from build123d import *

# Parameters (mm, degrees)
F0_R          = 4
F1_DEPTH      = 24.95
F2_W          = 40
F2_H          = 20
F3_DEPTH      = 150
F3_DEPTH_BACK = 150
F4_R          = 20
F5_DEPTH      = 50


with BuildPart() as f1:
    # F0 (on Top) → F1 (new body)
    with BuildSketch(Plane.XY):
        with BuildLine():
            Line((58.181364, 29.598313), (-78.941487, 29.598313))
            ThreePointArc((-78.941487, 29.598313), (-83.494247, 27.712498), (-85.380062, 23.159739))
            Line((-85.380062, 23.159739), (-85.380062, -34.03374))
            ThreePointArc((-85.380062, -34.03374), (-83.514933, -38.536559), (-79.012115, -40.401687))
            Line((-79.012115, -40.401687), (-73.01646, -40.401687))
            Line((-73.01646, -40.401687), (-58.498297, -40.401687))
            Line((-58.498297, -40.401687), (-46.752002, -40.401687))
            Line((-46.752002, -40.401687), (-43.284619, -40.401687))
            Line((-43.284619, -40.401687), (26.715381, -40.401687))
            Line((26.715381, -40.401687), (29.210588, -40.401687))
            Line((29.210588, -40.401687), (54.838952, -40.401687))
            Line((54.838952, -40.401687), (60.120346, -40.401687))
            ThreePointArc((60.120346, -40.401687), (63.302038, -39.083787), (64.619938, -35.902095))
            Line((64.619938, -35.902095), (64.619938, 23.159739))
            ThreePointArc((64.619938, 23.159739), (62.734124, 27.712498), (58.181364, 29.598313))
        make_face()
        with Locations((-77.880062, -32.901687)):
            Circle(F0_R, mode=Mode.SUBTRACT)
        with Locations((57.119938, -32.901687)):
            Circle(F0_R, mode=Mode.SUBTRACT)
        with Locations((-77.880062, 22.098313)):
            Circle(F0_R, mode=Mode.SUBTRACT)
        with Locations((57.119938, 22.098313)):
            Circle(F0_R, mode=Mode.SUBTRACT)
        Polygon((-58.498297, -40.401687), (-73.01646, -40.401687), (-46.752002, -66.558582), (-46.752002, -40.401687), align=None)
        Polygon((29.210588, -67.972728), (54.838952, -40.401687), (29.210588, -40.401687), align=None)
        Polygon((-46.752002, -40.401687), (-46.752002, -66.558582), (-46.752002, -82.901687), (-46.752002, -90.401687), (-39.252002, -90.401687), (21.710588, -90.401687), (29.210588, -90.401687), (29.210588, -82.901687), (29.210588, -67.972728), (29.210588, -40.401687), (26.715381, -40.401687), (-43.284619, -40.401687), align=None)
        with Locations((-39.252002, -82.901687)):
            Circle(F0_R, mode=Mode.SUBTRACT)
        with Locations((21.710588, -82.901687)):
            Circle(F0_R, mode=Mode.SUBTRACT)
    extrude(amount=-F1_DEPTH)

    # F2 (on face) → F3 (cut, two sides)
    with BuildSketch(Plane.YZ.offset(64.619938)) as f3_sk:
        with Locations((-5.902329, -10)):
            Rectangle(F2_W, F2_H)
    extrude(amount=-F3_DEPTH, mode=Mode.SUBTRACT)
    extrude(f3_sk.sketch, amount=-F3_DEPTH_BACK, mode=Mode.SUBTRACT)

    # F4 (on face) → F5 (cut)
    with BuildSketch(Plane.XZ.offset(90.401687)):
        with Locations((-8.770707, 0)):
            Circle(F4_R)
    extrude(amount=-F5_DEPTH, mode=Mode.SUBTRACT)


solid = f1.part
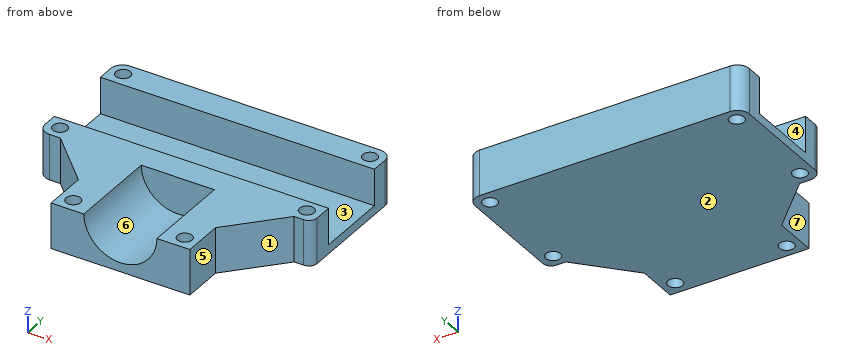
Verification items for the finished model (mm, model axes). Face numbers are marked on the shaded views. A direction names the side the tool comes from. Give positions to 0.01 mm unless a question says otherwise; leave off trailing zeros. Loops run counter-clockwise (first coordinate to the right, second up) from the corner with the lowest first, then second, coordinate; pieces in that order, holes last. Notation, with made-up numbers: (84, 55.25) - (99, 55.25) arc R16 cw to (99, 64.25) - close; hole circle Ø7 at (-25.75, 12.5). An arc over 180 degrees is marked (long way). Write item = value, one per line. Start each with the question number.
Q1. Thickness scan on line 1 (Y direction, x = 7, z = -18); line 2 (Y direction, x = -76, z = -7.25); line 3 (Y direction, x = -78.5, z = -20.75). Record the ranges inside material, lowest first.
Q2. Cross-section at C-C, the plane z = -23. Enter the section's corners in (x, y), and give its area (3 significant figures).
Q3. Depth check by flat-ended pin: P1, Ø6.5, axis at x = -39.25, y = -82.9, coming from the -Z side; P2, Ø2.5, axis at x = 57.5, z = -14, coming from the -Y side; P3, Ø4, axis at y = -48, z = -18.5, coming from the +X side; P4, Ø1.5, axis at y = -49, z = -11.5, coming from the -X side. Enter the tip coordinate at first touch or a pass-through.
Q4. Cross-section at B-B, the plane x = 16. Enter the section's corners in (y, z).
Q5. Tool access check on the marked faces 4, 5, 6 and 7. Record the directions out of +Z, -Z, +X, -X, +Y, -Y that give a thin tool (end or side, any length) a straight path to the whole face; none if there is none.
Q6. Cross-section at A-A, the plane z = -16. Enter the section's corners in (x, y), and give its area (3 significant figures).
Q7. Cross-section at D-D, the plane z = -6.5. Enter the section's corners in (x, y).
Q8. Mould release check, pull along Y, two halves, no side actions. Record for the marked faces 1, 2 and 3: released by +Y, released by -Y, zero draft, split by the parting line, or undercut.
Answer key:
q1.line_1 = -90.4 to -25.9, 14.1 to 29.6
q1.line_2 = -40.4 to -36.43, -29.37 to -25.9, 14.1 to 18.57, 25.63 to 29.6
q1.line_3 = -40.4 to -36.85, -28.95 to 18.15, 26.05 to 29.6
q2.outline = (-85.38, -34.03) arc R6.37 ccw to (-79.01, -40.4) - (-73.02, -40.4) - (-46.75, -66.56) - (-46.75, -90.4) - (29.21, -90.4) - (29.21, -67.97) - (54.84, -40.4) - (60.12, -40.4) arc R4.5 ccw to (64.62, -35.9) - (64.62, 23.16) arc R6.44 ccw to (58.18, 29.6) - (-78.94, 29.6) arc R6.44 ccw to (-85.38, 23.16) - close; hole circle Ø8 at (-77.88, -32.9); hole circle Ø8 at (-77.88, 22.1); hole circle Ø8 at (-39.25, -82.9); hole circle Ø8 at (21.71, -82.9); hole circle Ø8 at (57.12, -32.9); hole circle Ø8 at (57.12, 22.1)
q2.area = 14,700 mm^2
q3.P1 = through
q3.P2 = -40.4
q3.P3 = 49.64
q3.P4 = -65.14
q4.outline = (-90.4, -24.95) - (29.6, -24.95) - (29.6, 0) - (14.1, 0) - (14.1, -20) - (-25.9, -20) - (-25.9, 0) - (-90.4, 0) - close
q5.face_4 = +Z, +X, -X
q5.face_5 = +Z, -Z, +X, -Y
q5.face_6 = +Z, -Y
q5.face_7 = +Z, -Z, -X, -Y
q6.outline = (-85.38, -34.03) arc R6.37 ccw to (-79.01, -40.4) - (-73.02, -40.4) - (-46.75, -66.56) - (-46.75, -90.4) - (-20.77, -90.4) - (-20.77, -40.4) - (3.23, -40.4) - (3.23, -90.4) - (29.21, -90.4) - (29.21, -67.97) - (54.84, -40.4) - (60.12, -40.4) arc R4.5 ccw to (64.62, -35.9) - (64.62, -25.9) - (-85.38, -25.9) - close; (-85.38, 14.1) - (64.62, 14.1) - (64.62, 23.16) arc R6.44 ccw to (58.18, 29.6) - (-78.94, 29.6) arc R6.44 ccw to (-85.38, 23.16) - close; hole circle Ø8 at (-77.88, -32.9); hole circle Ø8 at (-77.88, 22.1); hole circle Ø8 at (-39.25, -82.9); hole circle Ø8 at (21.71, -82.9); hole circle Ø8 at (57.12, -32.9); hole circle Ø8 at (57.12, 22.1)
q6.area = 7,460 mm^2
q7.outline = (-85.38, -34.03) arc R6.37 ccw to (-79.01, -40.4) - (-73.02, -40.4) - (-46.75, -66.56) - (-46.75, -90.4) - (-27.68, -90.4) - (-27.68, -40.4) - (10.14, -40.4) - (10.14, -90.4) - (29.21, -90.4) - (29.21, -67.97) - (54.84, -40.4) - (60.12, -40.4) arc R4.5 ccw to (64.62, -35.9) - (64.62, -25.9) - (-85.38, -25.9) - close; (-85.38, 14.1) - (64.62, 14.1) - (64.62, 23.16) arc R6.44 ccw to (58.18, 29.6) - (-78.94, 29.6) arc R6.44 ccw to (-85.38, 23.16) - close; hole circle Ø8 at (-77.88, -32.9); hole circle Ø8 at (-77.88, 22.1); hole circle Ø8 at (-39.25, -82.9); hole circle Ø8 at (21.71, -82.9); hole circle Ø8 at (57.12, -32.9); hole circle Ø8 at (57.12, 22.1)
q8.face_1 = released by -Y
q8.face_2 = zero draft
q8.face_3 = undercut
